Part print with two shaded views. Sizes in mm from the minimum x, y, z corner. A direction names the side the tool comes from. Give positions to 0.01 mm unless a question says otherwise; leave off trailing zeros. Write each loop counter-clockwise with the first axis right and the second up, starting at its lowest first coordinate (ties: lowest second). Pieces come first, ordered by that corner, then holes. Notation, with made-up numbers: (36.25, -22.75) -> (56.25, -22.75) arc R19 ccw to (56.25, -17.75) -> close; hole circle Ø4 at (8, 13). An arc over 180 degrees is marked (long way). Write item = value, one per line. Start each with the question number.
Q1. Mould opens along Y. For the marked faces 1, 2 and 3 say: pulls with the +Y half, pulls with the -Y half, needs draft (parallel to the pull), parting line crosses it, or undercut.
Q2. Saw through at A-A, the plane y = 12.7. Give the number of separate pieces and of enclosed holes in the cut face, then the cut area to 3 significant figures.
Q3. Wall check: line 1 (Y direction, x = 12.7, z = 24.35); line 2 (X direction, y = 2, z = 17.25) (1 decimal); line 3 (Y direction, x = 13.75, z = 23). Give the ranges that are in metal, low to high.
Q4. Drop flat-ended pins along their axis: P1, Ø8, axis at y = 19, z = 16, coming from the +X side (1 decimal); P2, Ø12.5, axis at x = 9, y = 11.5, coming from the -Z side (1 decimal); P3, Ø6, axis at x = 5, y = 6.5, coming from the -Z side (1 decimal). Give the stop position or say it passes through.
Q5. Saw through at C-C, the plane x = 12.7. List the corners of the cut face in (y, z) (1 decimal).
Q6. Saw through at B-B, the plane z = 12.7. List the corners of the cut face in (x, y) (1 decimal).
Q7. Tool access for the marked faces 4 and 5: list every direction of +Z, -Z, +X, -X, +Y, -Y with a clear straight run to the whole face (end or side of a thin tool).
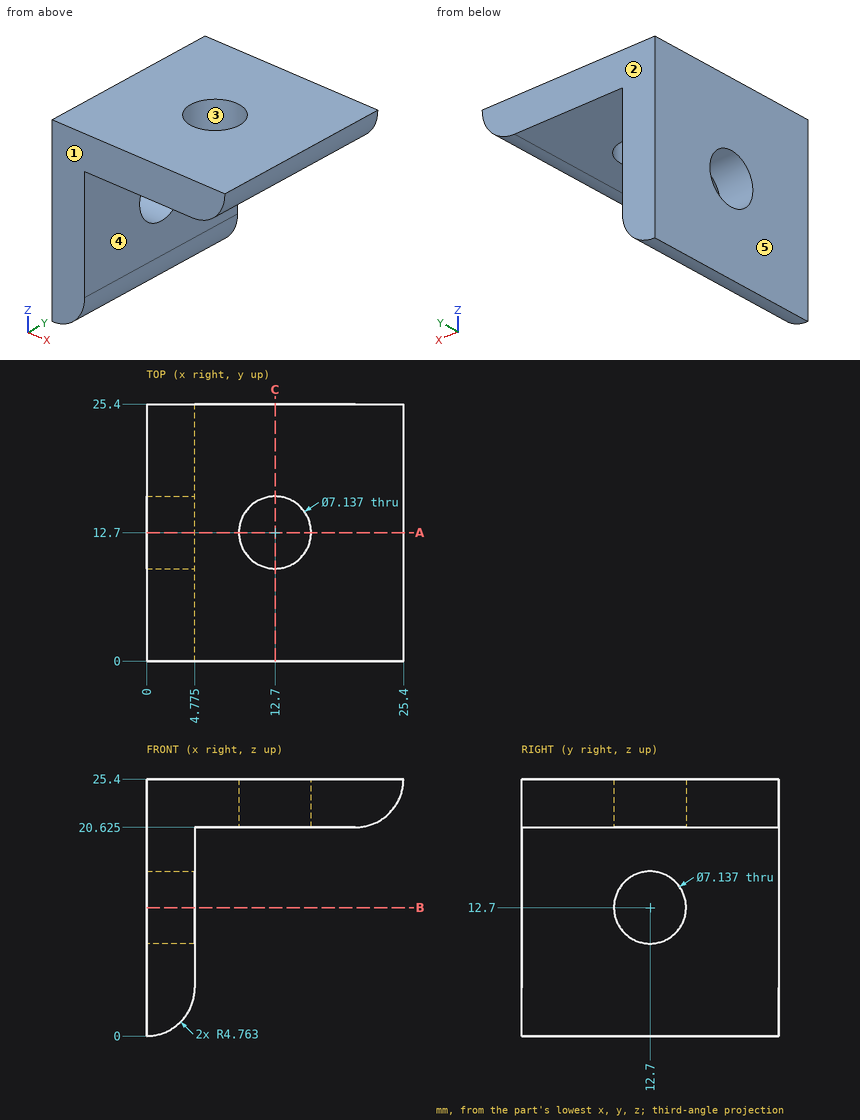
Report:
q1.face_1 = pulls with the -Y half
q1.face_2 = pulls with the +Y half
q1.face_3 = undercut
q2.separate_pieces = 3
q2.enclosed_holes = 0
q2.area = 142 mm2
q3.line_1 = 0 to 9.13, 16.27 to 25.4
q3.line_2 = 0 to 4.8
q3.line_3 = 0 to 9.29, 16.11 to 25.4
q4.P1 = 4.8
q4.P2 = 0.9
q4.P3 = 0.4
q5.outline = (0, 20.6) -> (9.1, 20.6) -> (9.1, 25.4) -> (0, 25.4) -> close; (16.3, 20.6) -> (25.4, 20.6) -> (25.4, 25.4) -> (16.3, 25.4) -> close
q6.outline = (0, 0) -> (4.8, 0) -> (4.8, 9.1) -> (0, 9.1) -> close; (0, 16.3) -> (4.8, 16.3) -> (4.8, 25.4) -> (0, 25.4) -> close
q7.face_4 = -Z, +X, +Y, -Y
q7.face_5 = +Z, -Z, -X, +Y, -Y
